Model file for the job. Use its own axes, mm. Face numbers are marked on the shaded views. A direction names the side the tool comes from. Give positions to 0.01 mm unless a question says otherwise; leave off trailing zeros. Write each loop counter-clockwise with the first axis right and the second up, starting at its lowest first coordinate (ties: lowest second). Pieces come first, ordered by that corner, then holes. Notation, with made-up numbers: M 20.5,83 L 76.5,83 A19 cw 76.5,88 Z; hole C 54.25,-39.5 d3. An arc over 180 degrees is marked long. Answer as a JSON object with one key per item and string values. Group by question number.
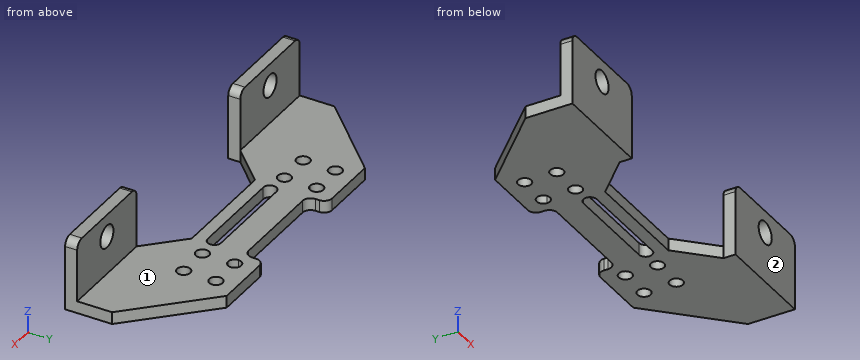
```python
from build123d import *

# Parameters (mm, degrees)
SKETCH_1_R          = 1.65
EXTRUDE_1_DEPTH     = 3
SKETCH_4_W          = 25.35
SKETCH_4_H          = 3
EXTRUDE_3_DEPTH     = 18
SKETCH_5_R          = 2.8
CUT_EXTRUDE_2_DEPTH = 18
FILLET_2_R          = 2


with BuildPart() as part:
    # 草图1 → 凸台-拉伸1 (new body)
    with BuildSketch(Plane.XY):
        Polygon((3.35, -13.65), (12, -5), (39, -5), (47.65, -13.65), (73, -13.65), (73, -5), (55, 13), (39, 13), (39, 8), (12, 8), (12, 13), (-4, 13), (-22, -5), (-22, -13.65), align=None)
        Circle(SKETCH_1_R, mode=Mode.SUBTRACT)
        with Locations((8, 0)):
            Circle(SKETCH_1_R, mode=Mode.SUBTRACT)
        with BuildLine():
            ThreePointArc((13.65, -1.975), (12, -0.325), (13.65, 1.325))
            Line((13.65, 1.325), (37.35, 1.325))
            ThreePointArc((37.35, 1.325), (39, -0.325), (37.35, -1.975))
            Line((37.35, -1.975), (13.65, -1.975))
        make_face(mode=Mode.SUBTRACT)
        with Locations((43, 0)):
            Circle(SKETCH_1_R, mode=Mode.SUBTRACT)
        with Locations((51, 0)):
            Circle(SKETCH_1_R, mode=Mode.SUBTRACT)
        with Locations((0, 8)):
            Circle(SKETCH_1_R, mode=Mode.SUBTRACT)
        with BuildLine():
            ThreePointArc((8, 6.35), (6.833273811, 9.166726189), (9.65, 8))
            ThreePointArc((9.65, 8), (9.166726189, 6.833273811), (8, 6.35))
        make_face(mode=Mode.SUBTRACT)
        with BuildLine():
            ThreePointArc((43, 6.35), (41.833273811, 6.833273811), (41.35, 8))
            ThreePointArc((41.35, 8), (44.166726189, 9.166726189), (43, 6.35))
        make_face(mode=Mode.SUBTRACT)
        with Locations((51, 8)):
            Circle(SKETCH_1_R, mode=Mode.SUBTRACT)
    extrude(amount=EXTRUDE_1_DEPTH)

    # 草图4 → 凸台-拉伸3 (add)
    with BuildSketch(Plane.XY):
        with Locations((-9.325, -15.15)):
            Rectangle(SKETCH_4_W, SKETCH_4_H)
        with Locations((60.325, -15.15)):
            Rectangle(SKETCH_4_W, SKETCH_4_H)
    extrude(amount=EXTRUDE_3_DEPTH)

    # 草图5 → 切除-拉伸2 (cut)
    with BuildSketch(Plane.XZ.offset(16.65)):
        with Locations(Location((60.325, 12.5, 0), (0, 0, 270))):
            Circle(SKETCH_5_R)
        with Locations(Location((-9.325, 12.5, 0), (0, 0, 270))):
            Circle(SKETCH_5_R)
    extrude(amount=-CUT_EXTRUDE_2_DEPTH, mode=Mode.SUBTRACT)

    # 圆角2
    fillet_2_edges = [part.edges().sort_by_distance(p)[0] for p in [
        (39, 13, 1.5),
        (12, 13, 1.5),
        (12, 8, 1.5),
        (39, 8, 1.5),
        (-22, -15.15, 18),
        (3.35, -15.15, 18),
        (47.65, -15.15, 18),
        (73, -15.15, 18),
    ]]
    fillet(fillet_2_edges, radius=FILLET_2_R)


solid = part.part
```
Q1. 3-axis set-ups, long thin cutter, end or side, ignore diameter. For the marked faces 1 and 2: which of +Z, -Z, +X, -X, +Y, -Y reach the whole face in a straight line?
Q2. Slice it at A-A, the plane x = 30. Write the cut outline in (y, z) (3 decimals), then the cut area to 3 significant figures.
Q3. Slice it at B-B, the plane x = 0. Write the cut outline in (y, z), then the cut area to 3 significant figures.
Q4. Drop flat-ended pins along their axis: P1, Ø3, axis at x = 0, y = 8, coming from the -Z side; P2, Ø2.5, axis at x = 25.5, z = 1, coming from the +Y side; P3, Ø0.5, axis at y = 10.5, z = 2, coming from the -X side; P4, Ø10, axis at x = 31, y = 6, coming from the -Z side. Give the stop position or say it passes through.
Q5. Wall check: L1, parallel to X at y = -15, z = 12.5 (3 decimals); L2, parallel to Y at x = 31, z = 2 (3 decimals). Give the ranges that are in metal, low to high.
Q6. Slice it at D-D, the plane y = 0. Write the cut outline in (x, z), then the cut area to 3 significant figures.
Q7. Slice it at C-C, the plane z = 12.5. Write the cut outline in (x, y) (3 decimals), then the cut area to 4 significant figures.
Solved:
{
 "1": {"face 1": "+Z, +X, -X, +Y", "face 2": "+Z, -Z, +X, -X, -Y"},
 "2": {"outline": "M -5,0 L -1.975,0 L -1.975,3 L -5,3 Z; M 1.325,0 L 8,0 L 8,3 L 1.325,3 Z", "area": "29.1 mm²"},
 "3": {"outline": "M -16.65,0 L -1.65,0 L -1.65,3 L -13.65,3 L -13.65,18 L -16.65,18 Z; M 1.65,0 L 6.35,0 L 6.35,3 L 1.65,3 Z; M 9.65,0 L 13,0 L 13,3 L 9.65,3 Z", "area": "114 mm²"},
 "4": {"P1": "passes through", "P2": "stops at y = 8", "P3": "stops at x = -6.75", "P4": "stops at z = 0"},
 "5": {"L1": "x = -22 to -12.125, -6.525 to 3.35, 47.65 to 57.525, 63.125 to 73", "L2": "y = -5 to -1.975, 1.325 to 8"},
 "6": {"outline": "M -17,0 L -1.65,0 L -1.65,3 L -17,3 Z; M 1.65,0 L 6.35,0 L 6.35,3 L 1.65,3 Z; M 9.65,0 L 12.03,0 L 12.03,3 L 9.65,3 Z; M 38.97,0 L 41.35,0 L 41.35,3 L 38.97,3 Z; M 44.65,0 L 49.35,0 L 49.35,3 L 44.65,3 Z; M 52.65,0 L 68,0 L 68,3 L 52.65,3 Z", "area": "135 mm²"},
 "7": {"outline": "M -22,-16.65 L -12.125,-16.65 L -12.125,-13.65 L -22,-13.65 Z; M -6.525,-16.65 L 3.35,-16.65 L 3.35,-13.65 L -6.525,-13.65 Z; M 47.65,-16.65 L 57.525,-16.65 L 57.525,-13.65 L 47.65,-13.65 Z; M 63.125,-16.65 L 73,-16.65 L 73,-13.65 L 63.125,-13.65 Z", "area": "118.5 mm²"}
}
